Drawing for the job (mm, zero at the part's lowest x, y, z). A direction names the side the tool comes from. Coordinates: 2 decimals unless noted, no trailing zeros. Write each loop counter-clockwise with the first axis right and the second up, starting at its lowest first coordinate (ties: lowest second). Pieces come first, ordered by that corner, then holes. Notation, with made-up numbers: M 56,74.25 L 100,74.25 A10 cw 100,90.25 Z; hole C 33,-27.75 d2. An arc over 180 degrees is marked long. Use a Markdown table: item, result. Add a question column.
Q1. Slice it at C-C on y = 50. Write the cut outline in (x, z), then the cut area to 3 significant figures.
Q2. Tool access for the marked faces 1, 2 and 3: list every direction of +Z, -Z, +X, -X, +Y, -Y with a clear straight run to the whole face (end or side of a thin tool).
Q3. Pin check, flat tips, straight feed: pin 1 Ø12.5 at (y, z) = (39.5, 9.5) entering from -X; pin 2 Ø12.5 at (x, z) = (77, 9) entering from +Y; pin 3 Ø23 at (x, y) = (24.49, 86.88) entering from -Z. Stop position of each tip, or through.
Q4. Wall check: L1, parallel to Y at x = 61, z = 13.5; L2, parallel to X at y = 84, z = 12.5; L3, parallel to X at y = 21.5, z = 23.25. Give the ranges that are in metal, low to high. Write a range as from..to.
Q5. Slice it at A-A on y = 91.5. Write the cut outline in (x, z).
Q6. Slice it at B-B on z = 6.5. Write the cut outline in (x, y) (1 decimal).
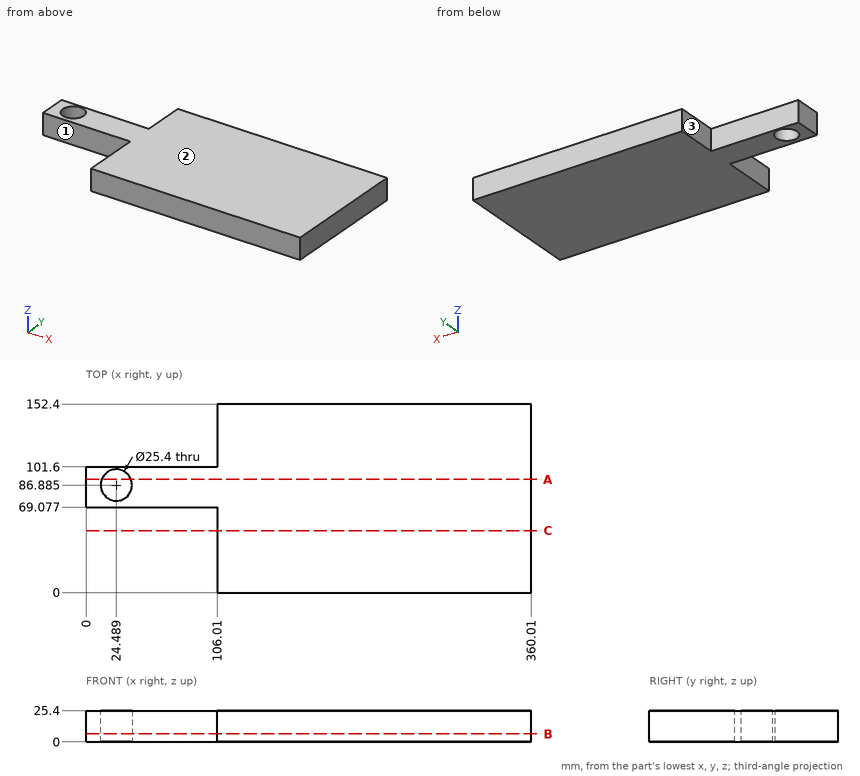
Recorded:
| question | item | result |
|---|---|---|
| 1 | outline | M 106.01,0 L 360.01,0 L 360.01,25.4 L 106.01,25.4 Z |
| 1 | area | 6,450 mm² |
| 2 | face 1 | +Z, -Z, -X, -Y |
| 2 | face 2 | +Z, +X, -X, +Y, -Y |
| 2 | face 3 | +Z, -Z, -X, +Y |
| 3 | pin 1 | x = 106.01 |
| 3 | pin 2 | y = 101.6 |
| 3 | pin 3 | through |
| 4 | L1 | 69.08..101.6 |
| 4 | L2 | 0..12.12, 36.86..360.01 |
| 4 | L3 | 106.01..360.01 |
| 5 | outline | M 0,0 L 12.66,0 L 12.66,25.4 L 0,25.4 Z; M 36.32,0 L 360.01,0 L 360.01,25.4 L 36.32,25.4 Z |
| 6 | outline | M 0,69.1 L 106,69.1 L 106,0 L 360,0 L 360,152.4 L 106,152.4 L 106,101.6 L 0,101.6 Z; hole C 24.5,86.9 d25.4 |
